```python
from build123d import *

# Parameters (mm, degrees)
BOSS_EXTRUDE1_DEPTH = 37.5
SKETCH2_W           = 14.5
SKETCH2_H           = 6
CUT_EXTRUDE1_DEPTH  = 1
SKETCH3_W           = 15
SKETCH3_H           = 2
SKETCH3_W_2         = 9
SKETCH3_H_2         = 7
CUT_EXTRUDE2_DEPTH  = 1


with BuildPart() as part:
    # Sketch1 → Boss-Extrude1 (new, symmetric)
    with BuildSketch(Plane(origin=(0, 0, 0), x_dir=(0, 0, -1), z_dir=(1, 0, 0))):
        with BuildLine():
            Line((-24.391141427, 5.424311485), (-25.309772394, -5.075688515))
            ThreePointArc((-25.309772394, -5.075688515), (-24.791937671, -6.601180415), (-23.317382998, -7.25))
            Line((-23.317382998, -7.25), (23.317382998, -7.25))
            ThreePointArc((23.317382998, -7.25), (24.791937671, -6.601180415), (25.309772394, -5.075688515))
            Line((25.309772394, -5.075688515), (24.391141427, 5.424311485))
            ThreePointArc((24.391141427, 5.424311485), (23.749932446, 6.724554674), (22.398752031, 7.25))
            Line((22.398752031, 7.25), (-22.398752031, 7.25))
            ThreePointArc((-22.398752031, 7.25), (-23.749932446, 6.724554674), (-24.391141427, 5.424311485))
        make_face()
    extrude(amount=BOSS_EXTRUDE1_DEPTH, both=True)

    # Sketch2 → Cut-Extrude1 (cut)
    with BuildSketch(Plane(origin=(0, 2.15894237, 24.676824207), x_dir=(1, 0, 0), z_dir=(0, 0.08715574274765166, 0.9961946980917462))):
        with Locations((-19.5, -1.222157705)):
            Rectangle(SKETCH2_W, SKETCH2_H)
        with Locations((0, -1.222157705)):
            Rectangle(SKETCH2_W, SKETCH2_H)
        with Locations((19.5, -1.222157705)):
            Rectangle(SKETCH2_W, SKETCH2_H)
    extrude(amount=-CUT_EXTRUDE1_DEPTH, mode=Mode.SUBTRACT)

    # Sketch3 → Cut-Extrude2 (cut)
    with BuildSketch(Plane(origin=(0, 2.15894237, -24.676824207), x_dir=(-1, 0, 0), z_dir=(0, 0.08715574274765166, -0.9961946980917462))):
        with Locations((19.25, -2.222157705)):
            Rectangle(SKETCH3_W, SKETCH3_H)
        with Locations((-13, -1.992211852)):
            Rectangle(SKETCH3_W_2, SKETCH3_H_2)
    extrude(amount=-CUT_EXTRUDE2_DEPTH, mode=Mode.SUBTRACT)


solid = part.part
```
Design review of the part built by this model. Coordinates are the model's own, in mm. Coordinates: 2 decimals unless noted, no trailing zeros. Write each loop counter-clockwise with the first axis right and the second up, starting at its lowest first coordinate (ties: lowest second). Pieces come first, ordered by that corner, then holes. Notation, with made-up numbers: M 26.5,-30 L 40.5,-30 A16 cw 40.5,-5 Z; hole C 30.25,14 d11. An arc over 180 degrees is marked long. Answer as a JSON object with one key per item and string values.
Item 1: Add section D-D, the plane x = -23. Give the boundary of the cut face in (y, z).
Outcome:
{"outline": "M -7.25,-23.32 A2 ccw -5.08,-25.31 L -1.05,-24.96 L -1.14,-23.96 L 0.85,-23.79 L 0.94,-24.78 L 5.42,-24.39 A2 ccw 7.25,-22.4 L 7.25,22.4 A2 ccw 5.42,24.39 L 3.93,24.52 L 3.84,23.53 L -2.13,24.05 L -2.05,25.04 L -5.08,25.31 A2 ccw -7.25,23.32 Z"}
Item 2: Add section B-B, the plane y = 0. Give the boundary of the cut face in (x, z).
Outcome:
{"outline": "M -37.5,-24.87 L -26.75,-24.87 L -26.75,-23.86 L -11.75,-23.86 L -11.75,-24.87 L 8.5,-24.87 L 8.5,-23.86 L 17.5,-23.86 L 17.5,-24.87 L 37.5,-24.87 L 37.5,24.87 L 26.75,24.87 L 26.75,23.86 L 12.25,23.86 L 12.25,24.87 L 7.25,24.87 L 7.25,23.86 L -7.25,23.86 L -7.25,24.87 L -12.25,24.87 L -12.25,23.86 L -26.75,23.86 L -26.75,24.87 L -37.5,24.87 Z"}
Item 3: Wall thickness on probe 1 along Z at (x, y) = (-25, -5.5); probe 2 along Y at (x, z) = (-32, 23.5); probe 3 along Z at (x, y) = (34.5, 0.5): over which ranges is each line inside the solid? List them lowest first.
Outcome:
{"probe 1": "-25.3 to 25.3", "probe 2": "-7.24 to 6.92", "probe 3": "-24.82 to 24.82"}
Item 4: Add section C-C, the plane x = 27.5. Give the boundary of the cut face in (y, z).
Outcome:
{"outline": "M -7.25,-23.32 A2 ccw -5.08,-25.31 L 5.42,-24.39 A2 ccw 7.25,-22.4 L 7.25,22.4 A2 ccw 5.42,24.39 L -5.08,25.31 A2 ccw -7.25,23.32 Z"}
Item 5: Add section A-A, the plane x = 3.5. Give the boundary of the cut face in (y, z), and give its area (3 significant figures).
Outcome:
{"outline": "M -7.25,-23.32 A2 ccw -5.08,-25.31 L 5.42,-24.39 A2 ccw 7.25,-22.4 L 7.25,22.4 A2 ccw 5.42,24.39 L 3.93,24.52 L 3.84,23.53 L -2.13,24.05 L -2.05,25.04 L -5.08,25.31 A2 ccw -7.25,23.32 Z", "area": "712 mm²"}
Item 6: Draft analysis for pull direction X (two halves, no side actions). For faces 1 (the flat face through (-19.145, -0.128, -23.873)), 2 (the flat face through (0.525, 0.101, -24.857)), 3 (the flat face through (-37.5, 0, 0)), state which applies: pulls with the +X half, pulls with the -X half, needs draft (parallel to the pull), parting line crosses it, or undercut.
Outcome:
{"face 1": "undercut", "face 2": "needs draft", "face 3": "pulls with the -X half"}
